Verification items for this drawing (mm, ordinates from the low corner). Round coordinates to 2 decimals unless told otherwise and drop trailing zeros. Loops run counter-clockwise (first coordinate to the right, second up) from the corner with the lowest first, then second, coordinate; pieces in that order, holes last. Notation, with made-up numbers: M 16.5,32 L 22.5,32 A23 ccw 22.5,47 Z; hole C -32.75,-24 d2. An arc over 180 degrees is marked long. Write item = value, one per line. Start each with the question number.
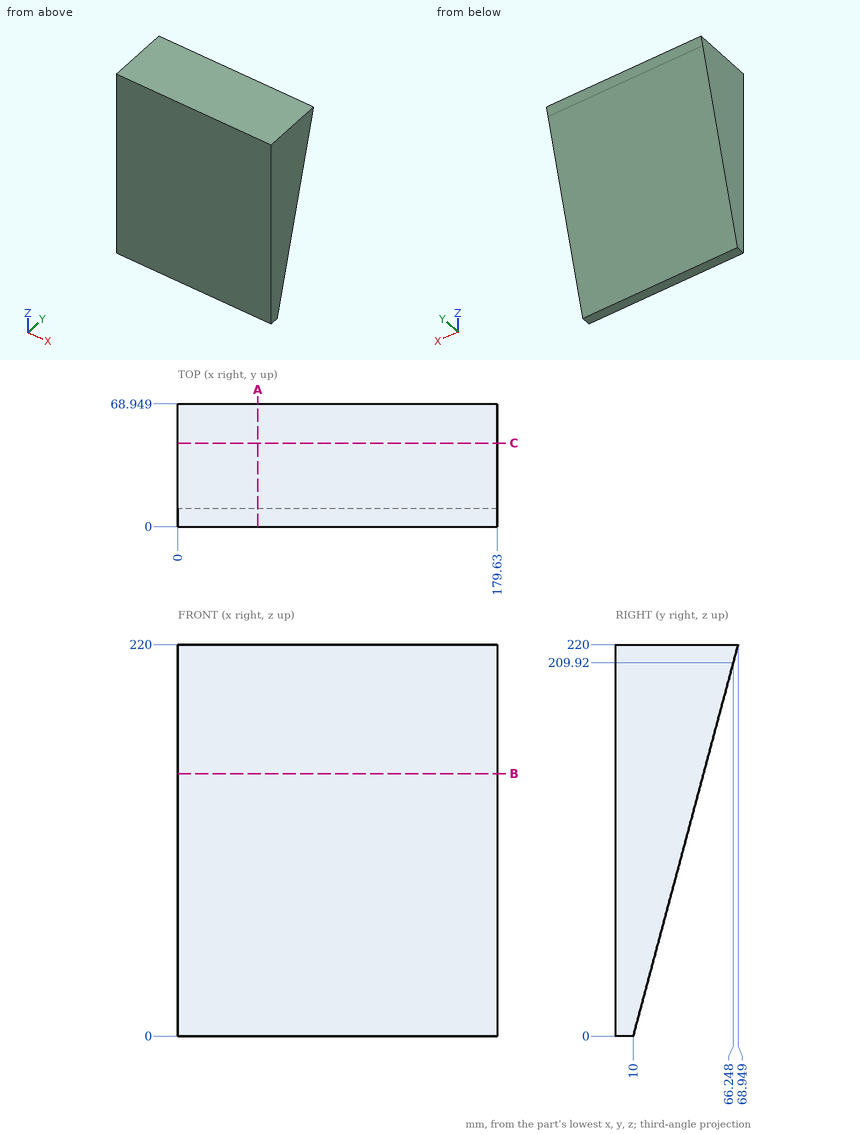
1. Section check B-B, the plane z = 147.5. Enter the section's corners in (x, y), and give its area (3 significant figures).
2. Section check C-C, the plane y = 47. Enter the section's corners in (x, z), and give its area (3 significant figures).
3. Thickness scan on line 1 (Y direction, x = 107, z = 143.5); line 2 (Y direction, x = 52, z = 41). Record the ranges inside material, lowest first.
4. Section check A-A, the plane x = 45. Enter the section's corners in (y, z), and give its area (3 significant figures).
5. Gauge pin test, flat ends, axial feed: P1, Ø4, axis at x = 100, z = 182, coming from the +Y side; P2, Ø12, axis at x = 142, z = 60, coming from the +Y side (1 decimal); P3, Ø5, axis at x = 41, z = 39, coming from the +Y side. Record the tip position at first contact, or that the pin passes through.
Computed values:
q1.outline = M 0,0 L 179.63,0 L 179.63,49.52 L 0,49.52 Z
q1.area = 8,900 mm2
q2.outline = M 0,138.09 L 179.63,138.09 L 179.63,220 L 0,220 Z
q2.area = 14,700 mm2
q3.line_1 = 0 to 48.45
q3.line_2 = 0 to 20.99
q4.outline = M 0,0 L 10,0 L 68.95,220 L 0,220 Z
q4.area = 8,680 mm2
q5.P1 = 59.3
q5.P2 = 27.7
q5.P3 = 21.12
